Build history of the part. All positions in model axes, mm. A direction names the side the tool comes from. Give positions to 0.01 mm unless a question says otherwise; leave off trailing zeros. Order: outer loops, then holes, each group sorted by start corner. A loop starts at its lowest first (then second) coordinate and runs counter-clockwise, first axis right, second up. Notation, with made-up numbers: (34, 0.25) - (93, 0.25) arc R12 ccw to (93, 17.25) - close; hole circle Ø5 at (62.5, 70.25). An arc over 180 degrees is marked (long way). Use a Markdown table: item, result. Add a question column.
(1) Flat gauge pins, fed straight in: pin 1 (10 mm diameter, centred on x = 214, z = 6485.5, fed in from +Y); pin 2 (6.5 mm diameter, centred on y = 2389, z = 6582.5, fed in from -X); pin 3 (14.5 mm diameter, centred on x = -110.66, y = 3083.27, fed in from +Z); pin 4 (7.5 mm diameter, centred on x = -404.62, z = 6909.42, fed in from +Y). Where does each tip first touch, or does it go through?
(2) Slice it at C-C (y = 2606). Write the cut outline in (x, z).
(3) Which spindle directions (+Z, -Z, +X, -X, +Y, -Y) get a long thin tool onto all of the face, cutting with end or side? Do faces 1 (the face through (-402, 2395.97, 6581)), 2 (the face through (56, 2383.27, 6578)). Say none if no direction does.
(4) Slice it at A-A (z = 6584). Write the cut outline in (x, y).
(5) Slice it at D-D (x = -430). Write the cut outline in (y, z), then the cut area to 3 significant figures.
(6) Slice it at B-B (x = 154). Write the cut outline in (y, z).
(7) Wall check: line 1 (Z direction, x = 200, y = 2475); line 2 (Y direction, x = 52, z = 6916). Give the ranges that are in metal, low to high.
from build123d import *

# Parameters (mm, degrees)
SKETCH1_R           = 161.29
BOSS_EXTRUDE2_DEPTH = 161.29
SKETCH2_W           = 7814.056
SKETCH2_H           = 18415
SKETCH2_R           = 161.29
BOSS_EXTRUDE3_DEPTH = 322.58
SCALE1_SCALE        = 0.039370079


with BuildPart() as part:
    # Sketch1 → Boss-Extrude2 (new body)
    with BuildSketch(Plane.XY):
        with BuildLine():
            Line((-454.375060891, 21951.534316097), (-11061.850005226, 735.172410385))
            ThreePointArc((-11061.850005226, 735.172410385), (-11039.602, 240.922843055), (-10607.474944335, 0))
            Line((-10607.474944335, 0), (10607.474944335, 0))
            ThreePointArc((10607.474944335, 0), (11039.602, 240.922843055), (11061.850005226, 735.172410385))
            Line((11061.850005226, 735.172410385), (454.375060891, 21951.534316097))
            ThreePointArc((454.375060891, 21951.534316097), (0, 22232.361905711), (-454.375060891, 21951.534316097))
        make_face()
        with Locations((-564.515, 11684)):
            Circle(SKETCH1_R, mode=Mode.SUBTRACT)
        with Locations((-564.515, 14732)):
            Circle(SKETCH1_R, mode=Mode.SUBTRACT)
        with Locations((-564.515, 17780)):
            Circle(SKETCH1_R, mode=Mode.SUBTRACT)
        with Locations((564.515, 17780)):
            Circle(SKETCH1_R, mode=Mode.SUBTRACT)
        with Locations((564.515, 14732)):
            Circle(SKETCH1_R, mode=Mode.SUBTRACT)
        with Locations((564.515, 11684)):
            Circle(SKETCH1_R, mode=Mode.SUBTRACT)
    extrude(amount=BOSS_EXTRUDE2_DEPTH)

    # Sketch2 → Boss-Extrude3 (add)
    # profile 1 of 2: a face of its own
    with BuildSketch(Plane(origin=(0, 0, 0), x_dir=(-1, 0, 0), z_dir=(0, -1, 0))):
        with Locations((-6500.040944335, -9368.79)):
            Rectangle(SKETCH2_W, SKETCH2_H)
        with Locations(Location((-6500.040944335, -17580.61, 0), (0, 0, 90))):
            Circle(SKETCH2_R, mode=Mode.SUBTRACT)
        with Locations(Location((-6500.040944335, -10483.85, 0), (0, 0, 90))):
            Circle(SKETCH2_R, mode=Mode.SUBTRACT)
        with Locations(Location((-6500.040944335, -3387.09, 0), (0, 0, 90))):
            Circle(SKETCH2_R, mode=Mode.SUBTRACT)
    # profile 2 of 2: a face of its own
    with BuildSketch(Plane(origin=(0, 0, 0), x_dir=(-1, 0, 0), z_dir=(0, -1, 0))):
        with Locations((6902.015055665, -9368.79)):
            Rectangle(SKETCH2_W, SKETCH2_H)
        with Locations(Location((6902.015055665, -3387.09, 0), (0, 0, 90))):
            Circle(SKETCH2_R, mode=Mode.SUBTRACT)
        with Locations(Location((6902.015055665, -10483.85, 0), (0, 0, 90))):
            Circle(SKETCH2_R, mode=Mode.SUBTRACT)
        with Locations(Location((6902.015055665, -17580.61, 0), (0, 0, 90))):
            Circle(SKETCH2_R, mode=Mode.SUBTRACT)
    extrude(amount=-BOSS_EXTRUDE3_DEPTH)


with BuildPart() as part_1:
    # Scale1: scaled about (-138.333124058, 2480.944734198, 6472.075728879)
    add(part.part.scale(SCALE1_SCALE).moved(Location((-132.886938071, 2383.269744663, 6217.269597821))))


solid = part_1.part
Solution:
| question | item | result |
|---|---|---|
| 1 | pin 1 | y = 2395.97 |
| 1 | pin 2 | x = -558.44 |
| 1 | pin 3 | z = 6223.62 |
| 1 | pin 4 | through |
| 2 | outline | (-471.51, 6217.27) - (205.73, 6217.27) - (205.73, 6223.62) - (-471.51, 6223.62) - close |
| 3 | face 1 | +Z, +X, -X, +Y |
| 3 | face 2 | +Z, -Z, +X, -X, -Y |
| 4 | outline | (-558.44, 2383.27) - (-250.8, 2383.27) - (-250.8, 2395.97) - (-558.44, 2395.97) - close; (-30.8, 2383.27) - (276.84, 2383.27) - (276.84, 2395.97) - (-30.8, 2395.97) - close |
| 5 | outline | (2383.27, 6217.27) - (2689.02, 6217.27) - (2689.02, 6223.62) - (2395.97, 6223.62) - (2395.97, 6948.62) - (2383.27, 6948.62) - close |
| 5 | area | 11,100 mm2 |
| 6 | outline | (2383.27, 6217.27) - (2709.47, 6217.27) - (2709.47, 6223.62) - (2395.97, 6223.62) - (2395.97, 6948.62) - (2383.27, 6948.62) - close |
| 7 | line 1 | 6217.27 to 6223.62 |
| 7 | line 2 | 2383.27 to 2395.97 |
